```python
from build123d import *

# Parameters (mm, degrees)
F0_W     = 406.4
F0_H     = 304.8
F1_DEPTH = 25.4
F2_R     = 5.08
F3_R     = 25.4
F4_DEPTH = 19.05


with BuildPart() as f1:
    # F0 (on Top) → F1 (new body)
    with BuildSketch(Plane.XY):
        Rectangle(F0_W, F0_H)
    extrude(amount=-F1_DEPTH)

    # F2
    f2_edges = [f1.edges().sort_by_distance(p)[0] for p in [
        (0, -152.4, 0),
        (203.2, 0, 0),
        (0, 152.4, 0),
        (-203.2, 0, 0),
    ]]
    fillet(f2_edges, radius=F2_R)

    # F3 (on face) → F4 (cut)
    with BuildSketch(Plane(origin=(0, 0, -25.4), x_dir=(1, 0, 0), z_dir=(0, 0, -1))):
        with Locations((-140.338207, 89.538207)):
            Circle(F3_R)
        with Locations((140.338207, 89.538207)):
            Circle(F3_R)
        with Locations((-140.338207, -89.538207)):
            Circle(F3_R)
        with Locations((140.338207, -89.538207)):
            Circle(F3_R)
    extrude(amount=-F4_DEPTH, mode=Mode.SUBTRACT)


solid = f1.part
```
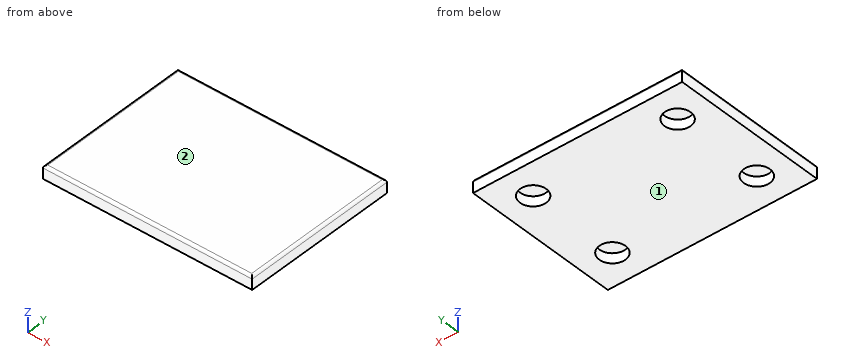
For this review, take the finished solid that the model builds, in its own axes (mm). Face numbers are marked on the shaded views. Coordinates: 2 decimals unless noted, no trailing zeros. Write each loop counter-clockwise with the first axis right and the second up, starting at its lowest first coordinate (ties: lowest second). Pieces come first, ordered by that corner, then holes.
(1) Add section B-B on z = -19. Give the boundary of the cut face in (x, y).
(2) Wall thickness on probe 1 along X at (y, z) = (91.5, -23.25); probe 2 along X at (y, z) = (104.5, -21.5); probe 3 along Y at (x, z) = (143, -22.25): over which ranges is each line inside the solid? List them lowest first.
(3) For pin 1 Ø15 at (x, y) = (136, 98.5) entering from -Z, flat-tipped, find the tip position at first contact; note if it passes through.
(4) Add section C-C on x = -140. Give the boundary of the cut face in (y, z), then the cut area to 3 significant figures.
(5) The part is to be moulded in two halves that separate along Z. For the marked faces 1 and 2, say which applies: +Z half, -Z half, draft (parallel to the pull), parting line (faces both ways), or undercut.
(6) Add section A-A on y = -70. Give the boundary of the cut face in (x, z).
Answer sheet:
1. outline: (-203.2, -152.4) - (203.2, -152.4) - (203.2, 152.4) - (-203.2, 152.4) - close; hole circle Ø50.8 at (-140.34, -89.54); hole circle Ø50.8 at (-140.34, 89.54); hole circle Ø50.8 at (140.34, -89.54); hole circle Ø50.8 at (140.34, 89.54)
2. probe 1: x = -203.2 to -165.66, -115.01 to 115.01, 165.66 to 203.2
2. probe 2: x = -203.2 to -160.86, -119.81 to 119.81, 160.86 to 203.2
2. probe 3: y = -152.4 to -114.8, -64.28 to 64.28, 114.8 to 152.4
3. pin 1: stops at z = -6.35
4. outline: (-152.4, -25.4) - (-114.94, -25.4) - (-114.94, -6.35) - (-64.14, -6.35) - (-64.14, -25.4) - (64.14, -25.4) - (64.14, -6.35) - (114.94, -6.35) - (114.94, -25.4) - (152.4, -25.4) - (152.4, -5.08) arc R5.08 ccw to (147.32, 0) - (-147.32, 0) arc R5.08 ccw to (-152.4, -5.08) - close
4. area: 5,800 mm2
5. face 1: -Z half
5. face 2: +Z half
6. outline: (-203.2, -25.4) - (-156.57, -25.4) - (-156.57, -6.35) - (-124.11, -6.35) - (-124.11, -25.4) - (124.11, -25.4) - (124.11, -6.35) - (156.57, -6.35) - (156.57, -25.4) - (203.2, -25.4) - (203.2, -5.08) arc R5.08 ccw to (198.12, 0) - (-198.12, 0) arc R5.08 ccw to (-203.2, -5.08) - close
